The listing builds one solid part. Answer for the finished solid, in the listing's coordinates (mm). Face numbers are marked on the shaded views. A direction names the side the tool comes from. Give positions to 0.01 mm unless a question says otherwise; leave off trailing zeros. Order: outer loops, then holes, each group sorted by start corner. A loop starts at its lowest first (then second) coordinate and runs counter-clockwise, first axis right, second up. Notation, with made-up numbers: (-6, 31.5) - (27, 31.5) arc R31 cw to (27, 59.5) - close; hole circle Ø9 at (81.25, -6). An arc over 180 degrees is marked (long way). Answer as CSV lines item,"result". Start each with the question number.
1. Flat-ended cylindrical pins translate along their axes: pin 1 (3 mm diameter, centred on x = 8, y = 0, fed in from -Z); pin 2 (3 mm diameter, centred on y = -6, z = -4, fed in from -X); pin 3 (2 mm diameter, centred on y = 5.5, z = -7, fed in from +X); pin 4 (4.5 mm diameter, centred on x = 7.5, y = 0.5, fed in from +Z). Find the tip coordinate at first contact, or state that the pin passes through.
2. Section A-A on x = 20 is taken. Give the vertices of the cut face in (y, z) (3 decimals).
3. Consider line 1 along Y through (x, z) = (8, -8) (3 decimals); line 2 along Z through (x, y) = (19.5, -4.25); line 3 along Y through (x, z) = (8, -5.6). Determine where each line is inside the solid, lowest interval first. Write a range as [from, to].
4. Section D-D on y = 0 is taken. Count the separate pieces of the cut face and the enclosed holes in it, and give its area (3 significant figures).
5. Section C-C on x = 30 is taken. Give the vertices of the cut face in (y, z) (3 decimals), and give its area (3 significant figures).
6. Which of the six approach directions +Z, -Z, +X, -X, +Y, -Y give full straight-line access (tool end or side, diameter ignored) to the marked faces 1, 2 and 3?
7. Section B-B on z = -4.4 is taken. Give the vertices of the cut face in (x, y) (3 decimals), and give its area (3 significant figures).
8. Determine the mould class of the marked faces 4, 5 and 6 for opening direction Y: +Y half, -Y half, draft (parallel to the pull), parting line (faces both ways), or undercut.
from build123d import *

# Parameters (mm, degrees)
BOSS_EXTRUDE1_START     = -9
SKETCH1_W               = 30
SKETCH1_H               = 12
BOSS_EXTRUDE1_DEPTH     = 5
BOSS_EXTRUDE2_START     = -9
SKETCH2_R               = 9
BOSS_EXTRUDE2_DEPTH     = 5
BOSS_EXTRUDE3_START     = -9
SKETCH3_R               = 6.5
BOSS_EXTRUDE3_DEPTH     = 5
CUT_EXTRUDE1_DEPTH      = 39.655530005
CUT_EXTRUDE1_DEPTH_BACK = 39.655530005
SKETCH4_R               = 3.25
CUT_EXTRUDE2_DEPTH      = 39.655530005
CUT_EXTRUDE2_DEPTH_BACK = 39.655530005
SKETCH5_R               = 1.725
CUT_EXTRUDE3_START      = -6.2
SKETCH6_R               = 2.9
CUT_EXTRUDE3_DEPTH      = 2.2
CUT_EXTRUDE4_START      = -6.2
SKETCH7_R               = 2.9
CUT_EXTRUDE4_DEPTH      = 2.2
CUT_EXTRUDE5_START      = -9
SKETCH8_R               = 2.9
CUT_EXTRUDE5_DEPTH      = 2.2
BOSS_EXTRUDE4_START     = -4
SKETCH9_R               = 3.5
BOSS_EXTRUDE4_DEPTH     = 1
CUT_EXTRUDE6_DEPTH      = 39.655530005
CUT_EXTRUDE6_DEPTH_BACK = 39.655530005
SKETCH10_R              = 1.725


with BuildPart() as part:
    # Sketch1 → Boss-Extrude1 (new body)
    with BuildSketch(Plane.XY.offset(BOSS_EXTRUDE1_START)):
        with Locations((15, 0)):
            Rectangle(SKETCH1_W, SKETCH1_H)
    extrude(amount=BOSS_EXTRUDE1_DEPTH)

    # Sketch2 → Boss-Extrude2 (add)
    with BuildSketch(Plane.XY.offset(BOSS_EXTRUDE2_START)):
        Circle(SKETCH2_R)
    extrude(amount=BOSS_EXTRUDE2_DEPTH)

    # Sketch3 → Boss-Extrude3 (add)
    with BuildSketch(Plane.XY.offset(BOSS_EXTRUDE3_START)):
        with Locations((30, 0)):
            Circle(SKETCH3_R)
    extrude(amount=BOSS_EXTRUDE3_DEPTH)

    # Sketch4 → Cut-Extrude1 (cut, two sides: drawn at the far end of the back side and taken through both)
    with BuildSketch(Plane.XY.offset(-CUT_EXTRUDE1_DEPTH_BACK)):
        Circle(SKETCH4_R)
    extrude(amount=CUT_EXTRUDE1_DEPTH + CUT_EXTRUDE1_DEPTH_BACK, mode=Mode.SUBTRACT)

    # Sketch5 → Cut-Extrude2 (cut, two sides: drawn at the far end of the back side and taken through both)
    with BuildSketch(Plane.XY.offset(-CUT_EXTRUDE2_DEPTH_BACK)):
        with Locations((8, 0)):
            Circle(SKETCH5_R)
        with Locations((20, 0)):
            Circle(SKETCH5_R)
        with Locations((30, 0)):
            Circle(SKETCH5_R)
    extrude(amount=CUT_EXTRUDE2_DEPTH + CUT_EXTRUDE2_DEPTH_BACK, mode=Mode.SUBTRACT)

    # Sketch6 → Cut-Extrude3 (cut)
    with BuildSketch(Plane.XY.offset(CUT_EXTRUDE3_START)):
        with Locations((8, 0)):
            Circle(SKETCH6_R)
    extrude(amount=CUT_EXTRUDE3_DEPTH, mode=Mode.SUBTRACT)

    # Sketch7 → Cut-Extrude4 (cut)
    with BuildSketch(Plane.XY.offset(CUT_EXTRUDE4_START)):
        with Locations((20, 0)):
            Circle(SKETCH7_R)
    extrude(amount=CUT_EXTRUDE4_DEPTH, mode=Mode.SUBTRACT)

    # Sketch8 → Cut-Extrude5 (cut)
    with BuildSketch(Plane.XY.offset(CUT_EXTRUDE5_START)):
        with Locations((30, 0)):
            Circle(SKETCH8_R)
    extrude(amount=CUT_EXTRUDE5_DEPTH, mode=Mode.SUBTRACT)

    # Sketch9 → Boss-Extrude4 (add)
    with BuildSketch(Plane.XY.offset(BOSS_EXTRUDE4_START)):
        with Locations((30, 0)):
            Circle(SKETCH9_R)
    extrude(amount=BOSS_EXTRUDE4_DEPTH)

    # Sketch10 → Cut-Extrude6 (cut, two sides: drawn at the far end of the back side and taken through both)
    with BuildSketch(Plane.XY.offset(-CUT_EXTRUDE6_DEPTH_BACK)):
        with Locations((30, 0)):
            Circle(SKETCH10_R)
    extrude(amount=CUT_EXTRUDE6_DEPTH + CUT_EXTRUDE6_DEPTH_BACK, mode=Mode.SUBTRACT)


solid = part.part
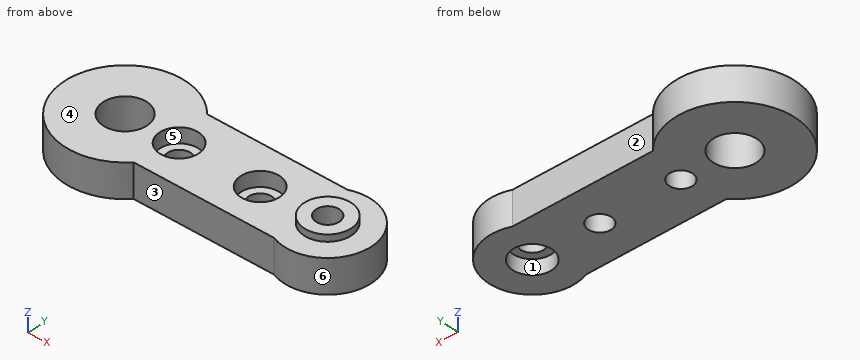
Checks:
1,pin 1,"passes through"
1,pin 2,"stops at x = -7.79"
1,pin 3,"stops at x = 34.69"
1,pin 4,"stops at z = -4"
2,outline,"(-6, -9) - (-1.725, -9) - (-1.725, -6.2) - (-2.9, -6.2) - (-2.9, -4) - (-6, -4) - close; (1.725, -9) - (6, -9) - (6, -4) - (2.9, -4) - (2.9, -6.2) - (1.725, -6.2) - close"
3,line 1,"y = [-6, -1.725], [1.725, 6]"
3,line 2,"z = [-9, -4]"
3,line 3,"y = [-6, -2.9], [2.9, 6]"
4,separate pieces,"5"
4,enclosed holes,"0"
4,area,"131 mm²"
5,outline,"(-6.5, -9) - (-2.9, -9) - (-2.9, -6.8) - (-1.725, -6.8) - (-1.725, -3) - (-3.5, -3) - (-3.5, -4) - (-6.5, -4) - close; (1.725, -6.8) - (2.9, -6.8) - (2.9, -9) - (6.5, -9) - (6.5, -4) - (3.5, -4) - (3.5, -3) - (1.725, -3) - close"
5,area,"46.1 mm²"
6,face 1,"-Z"
6,face 2,"+Z, -Z, +Y"
6,face 3,"+Z, -Z, -Y"
7,outline,"(6.708, -6) - (27.5, -6) arc R6.5 ccw (long way) to (27.5, 6) - (6.708, 6) arc R9 ccw (long way) to start; hole circle Ø6.5 at (0, 0); hole circle Ø5.8 at (8, 0); hole circle Ø5.8 at (20, 0); hole circle Ø3.45 at (30, 0)"
7,area,"488 mm²"
8,face 4,"draft"
8,face 5,"undercut"
8,face 6,"parting line"
